from build123d import *

# Parameters (mm, degrees)
ESQUISSE2_R                  = 5.5
BOSS_EXTRU_2_DEPTH           = 19
CHANFREIN1_SIZE              = 1.5
CHANFREIN1_SIZE2             = 7.5
ESQUISSE8_R                  = 4
BOSS_EXTRU_3_DEPTH           = 10.5
ESQUISSE9_R                  = 5.5
BOSS_EXTRU_4_DEPTH           = 10
ESQUISSE10_R                 = 3
BOSS_EXTRU_5_DEPTH           = 1
ESQUISSE12_R                 = 4
BOSS_EXTRU_6_DEPTH           = 10.5
CHANFREIN2_SIZE              = 1
ENL_V_MAT_EXTRU_1_DEPTH      = 52.58972766
ENL_V_MAT_EXTRU_1_DEPTH_BACK = 52.58972766
ESQUISSE15_R                 = 1.5


with BuildPart() as part:
    # Esquisse2 → Boss.-Extru.2 (new body)
    with BuildSketch(Plane(origin=(0, 0, 0), x_dir=(1, 0, 0), z_dir=(0, 1, 0))):
        with Locations(Location((0, 0, 0), (0, 0, 270))):
            Circle(ESQUISSE2_R)
    extrude(amount=BOSS_EXTRU_2_DEPTH)

    # Chanfrein1
    chanfrein1_edges = [part.edges().sort_by_distance(p)[0] for p in [
        (0, 0, -5.5),
    ]]
    chanfrein1_side = [part.faces().sort_by_distance(p)[0] for p in [
        (0, 0, 0),
    ]]
    chamfer(chanfrein1_edges, length=CHANFREIN1_SIZE, length2=CHANFREIN1_SIZE2, reference=chanfrein1_side[0])

    # Esquisse8 → Boss.-Extru.3 (add)
    with BuildSketch(Plane(origin=(0, 19, 0), x_dir=(1, 0, 0), z_dir=(0, 1, 0))):
        with Locations(Location((0, 0, 0), (0, 0, 90))):
            Circle(ESQUISSE8_R)
    extrude(amount=BOSS_EXTRU_3_DEPTH)

    # Esquisse9 → Boss.-Extru.4 (add)
    with BuildSketch(Plane(origin=(0, 29.5, 0), x_dir=(1, 0, 0), z_dir=(0, 1, 0))):
        with Locations(Location((0, 0, 0), (0, 0, 270))):
            Circle(ESQUISSE9_R)
    extrude(amount=BOSS_EXTRU_4_DEPTH)

    # Esquisse10 → Boss.-Extru.5 (add)
    with BuildSketch(Plane(origin=(0, 39.5, 0), x_dir=(1, 0, 0), z_dir=(0, 1, 0))):
        with Locations(Location((0, 0, 0), (0, 0, 270))):
            Circle(ESQUISSE10_R)
    extrude(amount=BOSS_EXTRU_5_DEPTH)

    # Esquisse12 → Boss.-Extru.6 (add)
    with BuildSketch(Plane(origin=(0, 40.5, 0), x_dir=(1, 0, 0), z_dir=(0, 1, 0))):
        with Locations(Location((0, 0, 0), (0, 0, 90))):
            Circle(ESQUISSE12_R)
    extrude(amount=BOSS_EXTRU_6_DEPTH)

    # Chanfrein2
    chanfrein2_edges = [part.edges().sort_by_distance(p)[0] for p in [
        (0, 51, 4),
    ]]
    chamfer(chanfrein2_edges, length=CHANFREIN2_SIZE)

    # Esquisse15 → Enlèv. mat.-Extru.1 (cut, two sides: drawn at the far end of the back side and taken through both)
    with BuildSketch(Plane.XY.offset(-ENL_V_MAT_EXTRU_1_DEPTH_BACK)):
        with Locations(Location((0, 42.5, 0), (0, 0, 90.000000025))):
            Circle(ESQUISSE15_R)
    extrude(amount=ENL_V_MAT_EXTRU_1_DEPTH + ENL_V_MAT_EXTRU_1_DEPTH_BACK, mode=Mode.SUBTRACT)


solid = part.part
The listing builds one solid part. Answer for the finished solid, in the listing's coordinates (mm). A direction names the side the tool comes from. Give positions to 0.01 mm unless a question says otherwise; leave off trailing zeros. Write each loop counter-clockwise with the first axis right and the second up, starting at its lowest first coordinate (ties: lowest second). Pieces come first, ordered by that corner, then holes. Notation, with made-up numbers: (84, -13) -> (114, -13) arc R26 ccw to (114, 23) -> close; hole circle Ø1 at (85.5, -19). An arc over 180 degrees is marked (long way). Use a Markdown table: item, result.
(1) Determine the mould class of faces 4 (the flat face through (0, 51, 0)), 5 (the conical face through (1.38, 2.97, 4.38)), 6 (the flat face through (-2, 19, -4)) for opening direction Y: released by +Y, released by -Y, zero draft, split by the parting line, or undercut.
Return value:
| item | result |
|---|---|
| face 4 | released by +Y |
| face 5 | released by -Y |
| face 6 | undercut |
(2) For faces 1 (the cylindrical face through (3.905, 45.184, 0.867)), 2 (the flat face through (-2, 29.5, -4)), 3 (the cylindrical face through (-5.37, 34.43, -1.19)), determine the directions among +Z, -Z, +X, -X, +Y, -Y from which every point of the face is accessible in a straight line to the end or side of a thin tool.
Return value:
| item | result |
|---|---|
| face 1 | +Y |
| face 2 | none |
| face 3 | +Y, -Y |
(3) Section C-C, the plane y = 4 is taken. Determine the outline of the cut face in (x, z).
Return value:
| item | result |
|---|---|
| outline | circle Ø9.6 at (0, 0) |
(4) Section A-A, the plane x = 0 is taken. Determine the outline of the cut face in (y, z).
Return value:
| item | result |
|---|---|
| outline | (0, -4) -> (7.5, -5.5) -> (19, -5.5) -> (19, -4) -> (29.5, -4) -> (29.5, -5.5) -> (39.5, -5.5) -> (39.5, -3) -> (40.5, -3) -> (40.5, -4) -> (41, -4) -> (41, 4) -> (40.5, 4) -> (40.5, 3) -> (39.5, 3) -> (39.5, 5.5) -> (29.5, 5.5) -> (29.5, 4) -> (19, 4) -> (19, 5.5) -> (7.5, 5.5) -> (0, 4) -> close; (44, -4) -> (50, -4) -> (51, -3) -> (51, 3) -> (50, 4) -> (44, 4) -> close |
(5) Flat-ended cylindrical pins translate along their axes: P1, Ø6, axis at y = 16, z = 2.5, coming from the -X side; P2, Ø5, axis at x = -3.5, y = 31.5, coming from the +Z side; P3, Ø1, axis at x = -2.5, y = 31.5, coming from the +Z side; P4, Ø4, axis at y = 32, z = -2.5, coming from the +X side. Find the tip coordinate at first contact, or state that the pin passes through.
Return value:
| item | result |
|---|---|
| P1 | x = -5.5 |
| P2 | z = 5.41 |
| P3 | z = 5.12 |
| P4 | x = 5.48 |
(6) Find the intervals of material crossed by probe 1 along Y at (x, z) = (0, -1.25); probe 2 along X at (y, z) = (42.5, 0.5); probe 3 along Y at (x, z) = (-0.75, -0.75), in increasing order. Write a range as from..to.
Return value:
| item | result |
|---|---|
| probe 1 | 0..41, 44..51 |
| probe 2 | -3.97..-1.5, 1.5..3.97 |
| probe 3 | 0..41.2, 43.8..51 |
(7) Section D-D, the plane y = 42.5 is taken. Determine the outline of the cut face in (x, z), then the cut area to 3 significant figures.
Return value:
| item | result |
|---|---|
| outline | (-1.5, -3.71) -> (-1.5, 3.71) arc R4 ccw to start; (1.5, -3.71) arc R4 ccw to (1.5, 3.71) -> close |
| area | 26.8 mm2 |
(8) Section B-B, the plane z = 0 is taken. Determine the outline of the cut face in (x, y), then the cut area to 3 significant figures.
Return value:
| item | result |
|---|---|
| outline | (-5.5, 7.5) -> (-4, 0) -> (4, 0) -> (5.5, 7.5) -> (5.5, 19) -> (4, 19) -> (4, 29.5) -> (5.5, 29.5) -> (5.5, 39.5) -> (3, 39.5) -> (3, 40.5) -> (4, 40.5) -> (4, 50) -> (3, 51) -> (-3, 51) -> (-4, 50) -> (-4, 40.5) -> (-3, 40.5) -> (-3, 39.5) -> (-5.5, 39.5) -> (-5.5, 29.5) -> (-4, 29.5) -> (-4, 19) -> (-5.5, 19) -> close; hole circle Ø3 at (0, 42.5) |
| area | 474 mm2 |
